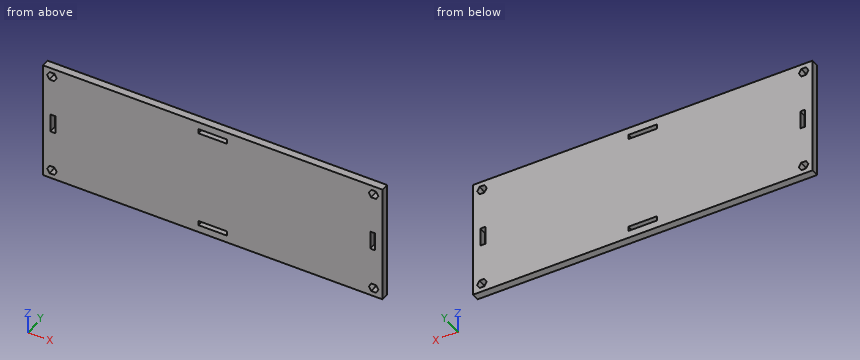
from build123d import *

# Parameters (mm, degrees)
CROQUIS1_W              = 180
CROQUIS1_H              = 64.5
SALIENTE_EXTRUIR1_DEPTH = 4
CROQUIS2_W              = 2.5
CROQUIS2_H              = 10
CORTAR_EXTRUIR1_DEPTH   = 4
MATRIZL1_COUNT          = 2
MATRIZL1_PITCH          = 169.5
CROQUIS3_W              = 15
CROQUIS3_H              = 2.5
CORTAR_EXTRUIR2_DEPTH   = 4
CORTAR_EXTRUIR3_DEPTH   = 4
MATRIZL2_COUNT          = 2
MATRIZL2_PITCH          = 170.52
MATRIZL2_COUNT_DIR2     = 2
MATRIZL2_PITCH_DIR2     = 55.1


with BuildPart() as part:
    # Croquis1 → Saliente-Extruir1 (new body)
    with BuildSketch(Plane(origin=(0, 0, 0), x_dir=(1, 0, 0), z_dir=(0, 1, 0))):
        Rectangle(CROQUIS1_W, CROQUIS1_H)
    extrude(amount=SALIENTE_EXTRUIR1_DEPTH)

    # Croquis2 → Cortar-Extruir1 (cut)
    with BuildSketch(Plane(origin=(0, 4, 0), x_dir=(1, 0, 0), z_dir=(0, 1, 0))):
        with Locations((84.75, 0)):
            Rectangle(CROQUIS2_W, CROQUIS2_H)
    cortar_extruir1 = extrude(amount=-CORTAR_EXTRUIR1_DEPTH, mode=Mode.SUBTRACT)

    # MatrizL1: Cortar-Extruir1 ×2
    with Locations(*[(-i * MATRIZL1_PITCH, 0, 0) for i in range(1, MATRIZL1_COUNT)]):
        add(cortar_extruir1, mode=Mode.SUBTRACT)

    # Croquis3 → Cortar-Extruir2 (cut)
    with BuildSketch(Plane(origin=(0, 0, 0), x_dir=(1, 0, 0), z_dir=(0, 1, 0))):
        with Locations((0, 27)):
            Rectangle(CROQUIS3_W, CROQUIS3_H)
        with Locations((0, -27)):
            Rectangle(CROQUIS3_W, CROQUIS3_H)
    extrude(amount=CORTAR_EXTRUIR2_DEPTH, mode=Mode.SUBTRACT)

    # Croquis4 → Cortar-Extruir3 (cut)
    with BuildSketch(Plane(origin=(0, 4, 0), x_dir=(1, 0, 0), z_dir=(0, 1, 0))):
        Polygon((-82.719317631, 27.55), (-83.989488223, 29.75), (-86.529829408, 29.75), (-87.8, 27.55), (-86.529829408, 25.35), (-83.989488223, 25.35), align=None)
    cortar_extruir3 = extrude(amount=-CORTAR_EXTRUIR3_DEPTH, mode=Mode.SUBTRACT)

    # MatrizL2: Cortar-Extruir3 2 × 2
    with Locations(*[(i * MATRIZL2_PITCH, 0, j * MATRIZL2_PITCH_DIR2) for i in range(MATRIZL2_COUNT) for j in range(MATRIZL2_COUNT_DIR2) if (i, j) != (0, 0)]):
        add(cortar_extruir3, mode=Mode.SUBTRACT)


solid = part.part
The listing builds one solid part. Answer for the finished solid, in the listing's coordinates (mm). Round coordinates to 2 decimals unless told otherwise and drop trailing zeros. Order: outer loops, then holes, each group sorted by start corner. A loop starts at its lowest first (then second) coordinate and runs counter-clockwise, first axis right, second up. Notation, with made-up numbers: (-26.5, -21) - (-16.5, -21) arc R29 ccw to (-16.5, 17) - close; hole circle Ø11 at (-27, 80). An arc over 180 degrees is marked (long way). Write item = value, one per line. Start each with the question number.
1) Straight lines are drawn through the part: L1, parallel to X at y = 2.95, z = -4.5; L2, parallel to Z at x = -5, y = 2.4; L3, parallel to X at y = 0.5, z = 27. For each, find the intervals that lie inside material, in ascending order.
2) Section A-A, the plane x = 2.5 is taken. Write down the section's boundary in (y, z), plus the area to 3 significant figures.
3) Section C-C, the plane y = 0.75 is taken. Count the separate pieces of the cut face and the enclosed holes in it, plus the area to 3 significant figures.
4) Section B-B, the plane z = 0.5 is taken. Write down the section's boundary in (x, y), plus the area to 3 significant figures.
Results list:
q1.L1 = -90 to -86, -83.5 to 83.5, 86 to 90
q1.L2 = -32.25 to -28.25, -25.75 to 25.75, 28.25 to 32.25
q1.L3 = -90 to -87.48, -83.04 to -7.5, 7.5 to 83.04, 87.48 to 90
q2.outline = (0, -32.25) - (4, -32.25) - (4, -28.25) - (0, -28.25) - close; (0, -25.75) - (4, -25.75) - (4, 25.75) - (0, 25.75) - close; (0, 28.25) - (4, 28.25) - (4, 32.25) - (0, 32.25) - close
q2.area = 238 mm^2
q3.separate_pieces = 1
q3.enclosed_holes = 8
q3.area = 11,400 mm^2
q4.outline = (-90, 0) - (-86, 0) - (-86, 4) - (-90, 4) - close; (-83.5, 0) - (83.5, 0) - (83.5, 4) - (-83.5, 4) - close; (86, 0) - (90, 0) - (90, 4) - (86, 4) - close
q4.area = 700 mm^2
